```python
from build123d import *

# Parameters (mm, degrees)
BOSS_EXTRUDE2_DEPTH                = 17.78
SKETCH2_R                          = 6.7437
CUT_EXTRUDE1_DEPTH                 = 91.384393011
SKETCH3_R                          = 11.938
CUT_EXTRUDE2_DEPTH                 = 1.016
BOSS_EXTRUDE3_DEPTH                = 19.05
BOSS_EXTRUDE3_DEPTH_BACK           = 19.05
SKETCH9_R                          = 12.7
CUT_EXTRUDE5_DEPTH                 = 130.70690942
F_1_8_0_125_DIAMETER_HOLE14_REACH  = 117.235
F_1_8_0_125_DIAMETER_HOLE14_BORE_R = 1.5875
FILLET1_R                          = 2.54


with BuildPart() as part:
    # Sketch1 → Boss-Extrude2 (new body)
    with BuildSketch(Plane(origin=(0, 0, 0), x_dir=(1, 0, 0), z_dir=(0, 1, 0))):
        with BuildLine():
            Line((-63.246, 22.032212417), (-10.16, 36.720354029))
            ThreePointArc((-10.16, 36.720354029), (0, 38.1), (10.16, 36.720354029))
            Line((10.16, 36.720354029), (63.246, 22.032212417))
            ThreePointArc((63.246, 22.032212417), (80.01, 0), (63.246, -22.032212417))
            Line((63.246, -22.032212417), (10.16, -36.720354029))
            ThreePointArc((10.16, -36.720354029), (0, -38.1), (-10.16, -36.720354029))
            Line((-10.16, -36.720354029), (-63.246, -22.032212417))
            ThreePointArc((-63.246, -22.032212417), (-80.01, 0), (-63.246, 22.032212417))
        make_face()
    extrude(amount=BOSS_EXTRUDE2_DEPTH)

    # Sketch2 → Cut-Extrude1 (cut, through all)
    with BuildSketch(Plane(origin=(0, 17.78, 0), x_dir=(1, 0, 0), z_dir=(0, 1, 0))):
        with Locations(Location((-57.15, 0, 0), (0, 0, 270))):
            Circle(SKETCH2_R)
    cut_extrude1 = extrude(amount=-CUT_EXTRUDE1_DEPTH, mode=Mode.SUBTRACT)

    # Sketch3 → Cut-Extrude2 (cut)
    with BuildSketch(Plane(origin=(0, 17.78, 0), x_dir=(1, 0, 0), z_dir=(0, 1, 0))):
        with Locations(Location((-57.15, 0, 0), (0, 0, 270))):
            Circle(SKETCH3_R)
    cut_extrude2 = extrude(amount=-CUT_EXTRUDE2_DEPTH, mode=Mode.SUBTRACT)

    # Mirror1: Cut-Extrude1, Cut-Extrude2 across plane
    add(cut_extrude1.mirror(Plane(origin=(0, 0, 0), x_dir=(0, 0, 1), z_dir=(1, 0, 0))), mode=Mode.SUBTRACT)
    add(cut_extrude2.mirror(Plane(origin=(0, 0, 0), x_dir=(0, 0, 1), z_dir=(1, 0, 0))), mode=Mode.SUBTRACT)

    # Sketch8 → Boss-Extrude3 (add, two sides)
    with BuildSketch(Plane(origin=(0, 0, 0), x_dir=(0, -1, 0), z_dir=(0.7071067811865464, 0, 0.7071067811865488))) as boss_extrude3_sk:
        with BuildLine():
            Line((-48.26, -25.4), (-17.78, -25.4))
            Line((-17.78, -25.4), (-17.78, 25.4))
            Line((-17.78, 25.4), (-48.26, 25.4))
            ThreePointArc((-48.26, 25.4), (-73.66, 0), (-48.26, -25.4))
        make_face()
    extrude(amount=BOSS_EXTRUDE3_DEPTH)
    extrude(boss_extrude3_sk.sketch, amount=-BOSS_EXTRUDE3_DEPTH_BACK)

    # Sketch9 → Cut-Extrude5 (cut, through all)
    with BuildSketch(Plane(origin=(13.470384182, 0, 13.470384182), x_dir=(0.7071067811865487, 0, -0.7071067811865465), z_dir=(0.7071067811865465, 0, 0.7071067811865487))):
        with Locations((0, 48.26)):
            Circle(SKETCH9_R)
    extrude(amount=-CUT_EXTRUDE5_DEPTH, mode=Mode.SUBTRACT)

    # 1/8 (0.125) Diameter Hole14 bore → 1/8 (0.125) Diameter Hole14 (cut, up to next)
    with BuildSketch(Plane(origin=(0, 73.66, 0), x_dir=(1, 0, 0), z_dir=(0, 1, 0)), mode=Mode.PRIVATE) as f_1_8_0_125_diameter_hole14_sk1:
        Circle(F_1_8_0_125_DIAMETER_HOLE14_BORE_R)
    f_1_8_0_125_diameter_hole14_tool1 = extrude(f_1_8_0_125_diameter_hole14_sk1.sketch, amount=-F_1_8_0_125_DIAMETER_HOLE14_REACH, mode=Mode.PRIVATE) & part.part
    add(f_1_8_0_125_diameter_hole14_tool1.solids().sort_by_distance((0, 73.66, 0))[0], mode=Mode.SUBTRACT)

    # Fillet1
    fillet1_edges = [part.edges().sort_by_distance(p)[0] for p in [
        (0, 17.78, 38.1),
        (36.703, 17.78, 29.376283223),
        (80.01, 17.78, 0),
        (36.703, 17.78, -29.376283223),
        (0, 17.78, -38.1),
        (-36.703, 17.78, -29.376283223),
        (-80.01, 17.78, 0),
        (4.490128061, 33.02, -31.430896424),
        (17.960512242, 17.78, -17.960512242),
        (-13.470384182, 17.78, -13.470384182),
        (-17.960512242, 17.78, 17.960512242),
        (-31.430896424, 33.02, 4.490128061),
        (-13.470384182, 73.66, -13.470384182),
        (31.430896424, 33.02, -4.490128061),
        (13.470384182, 73.66, 13.470384182),
        (-4.490128061, 33.02, 31.430896424),
        (13.470384182, 17.78, 13.470384182),
        (-36.703, 17.78, 29.376283223),
    ]]
    fillet(fillet1_edges, radius=FILLET1_R)


solid = part.part
```
Source: CAD feature listing. Evaluate the final solid. Frame: model axes, mm. A direction names the side the tool comes from. Round coordinates to 2 decimals unless told otherwise and drop trailing zeros. Write each loop counter-clockwise with the first axis right and the second up, starting at its lowest first coordinate (ties: lowest second). Pieces come first, ordered by that corner, then holes. Notation, with made-up numbers: M 82,1 L 103,1 A38 cw 103,39 Z; hole C 69,89.25 d7. An arc over 180 degrees is marked long. Answer as a JSON object with one key per item and string values. Group by question number.
(1) Section query A-A on y = 46.5. Output: boundary loops of the cut face in (x, z).
(2) Reachability of faces 1 (the cylindrical face through (-68.8, 17.3, -2.6)), 2 (the flat face through (-13.24, 34.79, -13.7)), 3 (the flat face through (18.12, 34.09, -17.8)), 4 (the cylindrical face through (30.38, 34.49, -4.46)) from +Z, -Z, +X, -X, +Y, -Y: full face, straight path, thin tool, end or side. Return the list, or none.
(3) First-contact query: pin 1 (12 mm diameter, centred on x = 56, z = -1, fed in from +Y); pin 2 (8 mm diameter, centred on x = -17.5, y = 9.5, fed in from -Z); pin 3 (4 mm diameter, centred on x = 10, y = 10, fed in from +Z); pin 4 (11 mm diameter, centred on x = -57.15, z = 0, fed in from +Y). Flat tips, straight axial feed; report the tip coordinate or a pass-through.
(4) Mould query, pull axis X, two halves, no side actions, for faces 5 (the cylindrical face through (-36.871, 17.056, 28.537)), 6 (the cylindrical face through (-50.464, 8.499, -0.878)), 7 (the cylindrical face through (36.1, 17.1, 28.7)). Classes: +X half, -X half, draft (parallel to the pull), parting line (faces both ways), or undercut.
(5) Ray query, line 1 (X direction, y = 7, z = 0); line 2 (X direction, y = 17, z = 0); line 3 (Y direction, x = -34.5, z = 10). Return the intervals inside material, ascending. Write a range as [from, to].
Computed values:
{
 "1": {"outline": "M -29.63,2.69 L -22.36,-4.58 L 4.58,22.36 L -2.69,29.63 A2.54 ccw -6.29,29.63 L -29.63,6.29 A2.54 ccw Z; M -4.58,-22.36 L 2.69,-29.63 A2.54 ccw 6.29,-29.63 L 29.63,-6.29 A2.54 ccw 29.63,-2.69 L 22.36,4.58 Z"},
 "2": {"face 1": "+Y", "face 2": "-Z, -X, +Y", "face 3": "-Z, +X, +Y", "face 4": "+X, +Y"},
 "3": {"pin 1": "y = 16.76", "pin 2": "z = -35.8", "pin 3": "z = 37.25", "pin 4": "through"},
 "4": {"face 5": "-X half", "face 6": "undercut", "face 7": "+X half"},
 "5": {"line 1": "[-80.01, -63.89], [-50.41, 50.41], [63.89, 80.01]", "line 2": "[-79.3, -69.09], [-45.21, 45.21], [69.09, 79.3]", "line 3": "[0, 17.78]"}
}
